Geometry: final body of the model. Coordinates: model frame, mm. A direction names the side the tool comes from. Give positions to 0.01 mm unless a question says otherwise; leave off trailing zeros. Loops run counter-clockwise (first coordinate to the right, second up) from the corner with the lowest first, then second, coordinate; pieces in that order, holes last. Notation, with made-up numbers: M 32.25,74.25 L 45.25,74.25 A5 cw 45.25,83.25 Z; hole C -24,35.25 d11. An arc over 180 degrees is marked long. Put each result on its own line as item: value.
```python
from build123d import *

# Parameters (mm, degrees)
SKETCH1_R           = 40
BOSS_EXTRUDE1_DEPTH = 70
BOSS_EXTRUDE1_TAPER = -10
CUT_EXTRUDE1_REACH  = 99.343
CUT_EXTRUDE1_START  = -45
SKETCH2_R           = 9
SKETCH3_R           = 7.5
BOSS_EXTRUDE2_DEPTH = 45
FILLET1_R           = 10
FILLET2_R           = 3


with BuildPart() as part:
    # Sketch1 → Boss-Extrude1 (new body)
    with BuildSketch(Plane(origin=(0, 0, 0), x_dir=(1, 0, 0), z_dir=(0, 1, 0))):
        Circle(SKETCH1_R)
    extrude(amount=BOSS_EXTRUDE1_DEPTH, taper=BOSS_EXTRUDE1_TAPER)

    # Sketch2 → Cut-Extrude1 (cut, up to next)
    with BuildSketch(Plane(origin=(0, 0, 0), x_dir=(0, 0, -1), z_dir=(1, 0, 0)).offset(CUT_EXTRUDE1_START), mode=Mode.PRIVATE) as cut_extrude1_sk1:
        with Locations((0, 42.296816006)):
            Circle(SKETCH2_R)
    cut_extrude1_tool1 = extrude(cut_extrude1_sk1.sketch, amount=-CUT_EXTRUDE1_REACH, mode=Mode.PRIVATE) & part.part
    add(cut_extrude1_tool1.solids().sort_by_distance((-45, 42.296816, 0))[0], mode=Mode.SUBTRACT)

    # Sketch3 → Boss-Extrude2 (add)
    with BuildSketch(Plane(origin=(0, 70, 0), x_dir=(1, 0, 0), z_dir=(0, 1, 0))):
        Circle(SKETCH3_R)
    extrude(amount=BOSS_EXTRUDE2_DEPTH)

    # Fillet1
    fillet1_edges = [part.edges().sort_by_distance(p)[0] for p in [
        (-40, 0, 0),
    ]]
    fillet(fillet1_edges, radius=FILLET1_R)

    # Fillet2
    fillet2_edges = [part.edges().sort_by_distance(p)[0] for p in [
        (-52.34288865, 70, 0),
    ]]
    fillet(fillet2_edges, radius=FILLET2_R)


solid = part.part
```
Item 1: Pin query (flat end, axial travel): pin 1 Ø4 at (x, y) = (21.5, 24.5) entering from -Z; pin 2 Ø2 at (y, z) = (27, 22.5) entering from -X; pin 3 Ø3 at (y, z) = (33.5, -13.5) entering from -X. Return the tip coordinate at first contact, or that it passes through.
Output values:
pin 1: z = -39.88
pin 2: x = -39.29
pin 3: x = -44.39
Item 2: Set-up query: faces 4 (the cylindrical face through (-7.493, 92.185, -0.33)), 5 (the conical face through (42.05, 31.31, 17.43)), 6 (the cylindrical face through (-46.54, 51.22, 1.17)). Return all of +Z, -Z, +X, -X, +Y, -Y with unobstructed straight access to the full face (end or side cutting, diameter ignored); none if empty.
Output values:
face 4: +Y
face 5: -Y
face 6: -X
Item 3: Section D-D on y = 45. Output: boundary loops of the cut face in (x, z).
Output values:
outline: M -47.16,-8.58 A47.93 ccw long -47.16,8.58 L -45,8.58 L -45,-8.58 Z
Item 4: Line query: probe 1 along Y at (x, z) = (-26, -17); probe 2 along Y at (x, z) = (-47, 0); probe 3 along X at (y, z) = (45.5, -32). Output: solid intervals per line, ascending. Write a range as [from, to].
Output values:
probe 1: [0, 70]
probe 2: [51.3, 70]
probe 3: [-35.81, 35.81]
Item 5: Section A-A on x = 0. Output: boundary loops of the cut face in (y, z), then the cut area to 3 significant figures.
Output values:
outline: M 0,-31.61 A10 ccw 8.26,-41.46 L 66.48,-51.72 A3 ccw 70,-48.77 L 70,-7.5 L 115,-7.5 L 115,7.5 L 70,7.5 L 70,48.77 A3 ccw 66.48,51.72 L 8.26,41.46 A10 ccw 0,31.61 Z
area: 7,110 mm²
Item 6: Mould query, pull axis Y, two halves, no side actions, for faces 1 (the flat face through (-1, 70, 10)), 2 (the flat face through (-45, 42, 0)), 3 (the flat face through (0, 0, 0)). Classes: pulls with the +Y half, pulls with the -Y half, needs draft (parallel to the pull), parting line crosses it, or undercut.
Output values:
face 1: pulls with the +Y half
face 2: undercut
face 3: pulls with the -Y half
Item 7: Section C-C on y = 29. Output: boundary loops of the cut face in (x, z).
Output values:
outline: C 0,0 d90.23
Item 8: Section B-B on y = 103. Output: boundary loops of the cut face in (x, z), then the cut area to 3 significant figures.
Output values:
outline: C 0,0 d15
area: 177 mm²
